Part model, mm, in its own coordinate system. A direction names the side the tool comes from. Round coordinates to 2 decimals unless told otherwise and drop trailing zeros. Write each loop counter-clockwise with the first axis right and the second up, starting at its lowest first coordinate (ties: lowest second). Pieces come first, ordered by that corner, then holes. Notation, with made-up numbers: M 31.25,27 L 66.25,27 A18 ccw 66.25,58 Z; hole C 5,11 d8. An arc over 180 degrees is marked long. Use a Markdown table: item, result. Add a question column.
1) Which spindle directions (+Z, -Z, +X, -X, +Y, -Y) get a long thin tool onto all of the face, cutting with end or side? Do faces 4 (the face through (-4, 0, -2)), 5 (the face through (20, 1.3, -1.3)), 6 (the face through (11, -3, 0)), 7 (the face through (-3.014, -1.293, 0.76)). Say none if no direction does.
2) Two-plate mould, pull along Z, no slides. Class faces 1 (the face through (-1.75, -0.59, 4.46)), 2 (the face through (-3.014, -1.305, -0.74)), 3 (the face through (27, 0, 0)): released by +Z, released by -Z, zero draft, split by the parting line, or undercut.
3) Wall check: probe 1 along Y at (x, z) = (21, 1); probe 2 along X at (y, z) = (1.5, -1.5); probe 3 along X at (y, z) = (-2, -3). Give the ranges that are in metal, low to high.
4) Drop flat-ended pins along their axis: P1, Ø5, axis at x = 7.5, z = -3.5, coming from the +Y side; P2, Ø1.5, axis at x = 5, y = 3, coming from the +Z side; P3, Ø0.9, axis at y = 0.5, z = -0.5, coming from the -X side; P4, Ø2.5, axis at y = 0, z = -2, coming from the +X side. Give the stop position or say it passes through.
5) Slice it at A-A on x = 11.5. Write the cut outline in (y, z).
Autodesk Inventor part; units mm, degrees
ref_plane "YZ Plane" through (0, 0, 0) normal (1, 0, 0) x (0, 1, 0)
ref_plane "XZ Plane" through (0, 0, 0) normal (0, 1, 0) x (-1, 0, 0)
ref_plane "XY Plane" through (0, 0, 0) normal (0, 0, 1) x (1, 0, 0)
sketch "Sketch_7" plane through (0, 0, 0) normal (0, 0, 1) x (1, 0, 0)
  line L0 (27, 0) -> (-1.134, 0)
  line L1 (-1.134, 0) -> (-2, 1.5)
  line L2 (-2, 1.5) -> (-4, 1.5)
  line L3 (-4, 1.5) -> (-4, 4.05)
  line L4 (-4, 4.05) -> (-3.55, 4.5)
  line L5 (-3.55, 4.5) -> (0, 4.5)
  line L6 (0, 4.5) -> (0, 3.25)
  arc A0 (0, 3.25) -> (0.7, 2.7) centre (0.5749, 3.2612) ccw
  line L7 (0.7, 2.7) -> (1, 3)
  line L8 (1, 3) -> (20, 3)
  line L9 (20, 3) -> (20, 1.5)
  line L10 (20, 1.5) -> (20.7, 1.5)
  line L11 (20.7, 1.5) -> (21.2, 2)
  line L12 (21.2, 2) -> (26.5705, 2)
  line L13 (26.5705, 2) -> (27, 1.5705)
  line L14 (27, 1.5705) -> (27, 0)
  line L15 (27, 0) -> (-1.134, 0)
revolve "Revolution1" add sketch "Sketch_7" angle 360 about axis through (27, 0, 0) along (1, 0, 0)
thread "Thread1"
sketch "Sketch_4" plane through (-4, 0, 0) normal (1, 0, 0) x (0, 0, -1)
  line L0 (-1.5, -0.866) -> (0, -1.7321)
  line L1 (0, -1.7321) -> (1.5, -0.866)
  line L2 (1.5, -0.866) -> (1.5, 0.866)
  line L3 (1.5, 0.866) -> (0, 1.7321)
  line L4 (0, 1.7321) -> (-1.5, 0.866)
  line L5 (-1.5, 0.866) -> (-1.5, -0.866)
extrude "Extrusion1" cut sketch "Sketch_4" along normal blind 2
properties part number "MSB6-20" material "鋼、炭素鋼"
Entries:
| question | item | result |
|---|---|---|
| 1 | face 4 | +Z, -Z, -X, +Y, -Y |
| 1 | face 5 | none |
| 1 | face 6 | +X |
| 1 | face 7 | -X |
| 2 | face 1 | split by the parting line |
| 2 | face 2 | undercut |
| 2 | face 3 | zero draft |
| 3 | probe 1 | y = -1.5 to 1.5 |
| 3 | probe 2 | x = -4 to 20 |
| 3 | probe 3 | x = -4 to 0 |
| 4 | P1 | stops at y = 2.83 |
| 4 | P2 | stops at z = 1.98 |
| 4 | P3 | stops at x = -1.8 |
| 4 | P4 | stops at x = 27 |
| 5 | outline | C 0,0 d6 |
